```python
from build123d import *

# Parameters (mm, degrees)
F1_DEPTH = 20
F2_W     = 20
F2_H     = 20
F3_DEPTH = 20


with BuildPart() as f1:
    # F0 (on Right) → F1 (new body)
    with BuildSketch(Plane.YZ):
        Polygon((43.928572, -20), (43.928572, 20), (23.928572, 20), (23.928572, 0), (3.928572, 0), (3.928572, -20), align=None)
    extrude(amount=F1_DEPTH)

    # F2 (on Right) → F3 (join)
    with BuildSketch(Plane.YZ):
        with Locations((33.10277, -10)):
            Rectangle(F2_W, F2_H)
    extrude(amount=-F3_DEPTH)


solid = f1.part
```
Geometry check sheet. Reference: the model listing, model coordinates, mm. A direction names the side the tool comes from. Round coordinates to 2 decimals unless told otherwise and drop trailing zeros. Loops run counter-clockwise (first coordinate to the right, second up) from the corner with the lowest first, then second, coordinate; pieces in that order, holes last. Notation, with made-up numbers: (16.25, 24) - (56.25, 24) arc R19 ccw to (56.25, 39) - close; hole circle Ø8 at (0, 67.5). An arc over 180 degrees is marked (long way). Write item = value, one per line. Start each with the question number.
1. Depth check by flat-ended pin: pin 1 (15.5 mm diameter, centred on y = 14.5, z = -14, fed in from -X); pin 2 (4 mm diameter, centred on x = 9.5, z = 13.5, fed in from -Y); pin 3 (16 mm diameter, centred on x = -7.5, z = -11.5, fed in from -Y); pin 4 (6 mm diameter, centred on x = -8, z = -13, fed in from +Y). Enter the tip coordinate at first touch or a pass-through.
2. Section check A-A on z = -7.5. Enter the section's corners in (x, y).
3. Thickness scan on line 1 (Y direction, x = -16.5, z = -3); line 2 (X direction, y = 11, z = -11.5); line 3 (Y direction, x = 16, z = 5). Record the ranges inside material, lowest first.
4. Section check B-B on y = 36. Enter the section's corners in (x, z).
5. Set-up check for faces 1 (the face through (-20, 33, -10)), 2 (the face through (-10, 23.103, -10)), 3 (the face through (-10, 43.103, -10)), 4 (the face through (10, 23.929, 10)), 5 (the face through (20, 28, -4)): record each of +Z, -Z, +X, -X, +Y, -Y from which the full face is reachable in a straight line by a thin tool's end or side.
6. Section check D-D on x = -11. Enter the section's corners in (y, z), then the cut area to 3 significant figures.
7. Section check C-C on x = 16.5. Enter the section's corners in (y, z), then the cut area to 3 significant figures.
Working result:
q1.pin_1 = 0
q1.pin_2 = 23.93
q1.pin_3 = 3.93
q1.pin_4 = 43.1
q2.outline = (-20, 23.1) - (0, 23.1) - (0, 3.93) - (20, 3.93) - (20, 43.93) - (0, 43.93) - (0, 43.1) - (-20, 43.1) - close
q3.line_1 = 23.1 to 43.1
q3.line_2 = 0 to 20
q3.line_3 = 23.93 to 43.93
q4.outline = (-20, -20) - (20, -20) - (20, 20) - (0, 20) - (0, 0) - (-20, 0) - close
q5.face_1 = +Z, -Z, -X, +Y, -Y
q5.face_2 = +Z, -Z, -X, -Y
q5.face_3 = +Z, -Z, -X, +Y
q5.face_4 = +Z, +X, -X, -Y
q5.face_5 = +Z, -Z, +X, +Y, -Y
q6.outline = (23.1, -20) - (43.1, -20) - (43.1, 0) - (23.1, 0) - close
q6.area = 400 mm^2
q7.outline = (3.93, -20) - (43.93, -20) - (43.93, 20) - (23.93, 20) - (23.93, 0) - (3.93, 0) - close
q7.area = 1,200 mm^2
